For this review, take the finished solid that the model builds, in its own axes (mm). Give positions to 0.01 mm unless a question says otherwise; leave off trailing zeros. Write each loop counter-clockwise with the first axis right and the second up, starting at its lowest first coordinate (ties: lowest second). Pieces come first, ordered by that corner, then holes. Notation, with made-up numbers: M -27.5,-13 L 17.5,-13 A14 cw 17.5,-1 Z; hole C 68.25,62.5 d6. An arc over 180 degrees is marked long. Answer as a JSON object with one key per item and string values. Group by question number.
Autodesk Inventor part; units mm, degrees
ref_plane "YZ Plane" through (0, 0, 0) normal (1, 0, 0) x (0, 1, 0)
ref_plane "XZ Plane" through (0, 0, 0) normal (0, 1, 0) x (-1, 0, 0)
ref_plane "XY Plane" through (0, 0, 0) normal (0, 0, 1) x (1, 0, 0)
sketch "スケッチ1" plane through (0, 0, 0) normal (0, 0, 1) x (1, 0, 0)
  circle A0 centre (0, 0) radius 67.5
  dimension "d0" = 135
extrude "プレート1" add sketch "スケッチ1" along normal blind 2
sketch "スケッチ2" plane through (0, 0, 2) normal (0, 0, 1) x (1, 0, 0)
  circle A0 centre (0, 0) radius 38.5
  dimension "d2" = 77
extrude "押し出し1" cut sketch "スケッチ2" against normal through all
sketch "スケッチ3" plane through (0, 0, 2) normal (0, 0, 1) x (1, 0, 0)
  circle A0 centre (0, 0) radius 62.5
  point P0 (16.1762, 60.3704)
  point P1 (-16.1762, 60.3704)
  point P2 (-44.1942, 44.1942)
  point P3 (-60.3704, 16.1762)
  point P4 (-60.3704, -16.1762)
  point P5 (-44.1942, -44.1942)
  point P6 (-16.1762, -60.3704)
  point P7 (16.1762, -60.3704)
  point P8 (44.1942, -44.1942)
  point P9 (60.3704, -16.1762)
  point P10 (60.3704, 16.1762)
  point P11 (44.1942, 44.1942)
  dimension "d5" = 125
  dimension "d8" = 360
  dimension "d36" = 0
hole "穴1" at (16.1762, 60.3704, 2) at (-16.1762, 60.3704, 2) at (-44.1942, 44.1942, 2) at (-60.3704, 16.1762, 2) at (-60.3704, -16.1762, 2) at (-44.1942, -44.1942, 2) at (-16.1762, -60.3704, 2) at (16.1762, -60.3704, 2) at (44.1942, -44.1942, 2) at (60.3704, -16.1762, 2) at (60.3704, 16.1762, 2) at (44.1942, 44.1942, 2) direction (0, 0, -1) diameter 4.5 end through all
sketch "スケッチ4" plane through (0, 0, 2) normal (0, 0, 1) x (1, 0, 0)
  circle A0 centre (0, 0) radius 49
  point P0 (-34.6482, 34.6482)
  point P1 (-34.6482, -34.6482)
  point P2 (34.6482, -34.6482)
  point P3 (34.6482, 34.6482)
  dimension "d17" = 98
  dimension "d20" = 360
  dimension "d29" = 0
hole "穴2" at (-34.6482, 34.6482, 2) at (-34.6482, -34.6482, 2) at (34.6482, -34.6482, 2) at (34.6482, 34.6482, 2) direction (0, 0, -1) diameter 4.5 end through all
sketch "スケッチ6" plane through (0, 0, 0) normal (0, 0, -1) x (-1, 0, 0)
  circle A0 centre (0, 0) radius 37.5
  line L0 (-4.75, -42.3) -> (4.75, -42.3)
  line L1 (-4.75, -37.5) -> (4.75, -37.5)
  circle A1 centre (0, -37.5) radius 4.8
  point P0 (-4.75, -51.1)
  point P1 (4.75, -51.1)
  dimension "d37" = 75
  dimension "d38" = 9.5
  dimension "d39" = 8.8
  dimension "d40" = 13.6
  dimension "d41" = 4.75
hole "穴3" at (4.75, -51.1, 0) at (-4.75, -51.1, 0) direction (0, 0, 1) diameter 2.4 end through all
equation "\"d15\" = Thickness"
equation "\"d27\" = Thickness"
equation "\"d47\" = Thickness"
equation "\"d1\" = Thickness"
equation "\"BendRadius\" = Thickness"
equation "\"BendReliefWidth\" = Thickness"
equation "\"BendReliefDepth\" = 0.5 * Thickness"
equation "\"CornerReliefSize\" = 4 * Thickness"
equation "\"MinimumRemnant\" = 2 * Thickness"
equation "\"TransitionRadius\" = BendRadius"
equation "\"JacobiRadiusSize\" = BendRadius"
equation "\"GapSize\" = Thickness"
properties part number "unit-j2-plate1" material "CFRP"
Item 1: Draft analysis for pull direction X (two halves, no side actions). For faces 1 (the cylindrical face through (-53.57, 41.07, 0.99)), 2 (the flat face through (29, -29, 2)), 3 (the cylindrical face through (15.5, 58.224, 0.986)), state which applies: released by +X, released by -X, zero draft, split by the parting line, or undercut.
Item 2: Consider section A-A (x = 0). Give the boundary of the cut face in (y, z), plus the area to 3 significant figures.
Item 3: Consider section D-D (y = 54). Give the boundary of the cut face in (x, z).
Item 4: To check wall thickness, follow probe 1 along X at (y, z) = (45.5, 0.45); probe 2 along X at (y, z) = (-51, 0.9); probe 3 along Y at (x, z) = (16, 1.35). State the ranges of each line that lie inside material, in increasing order.
Item 5: Consider section C-C (z = 1.5). State how many separate pieces and enclosed holes the cut face has, plus the area to 3 significant figures.
Item 6: Insertion check: P1, Ø6, axis at x = -44.19, y = 44.19, coming from the -Z side; P2, Ø2.5, axis at x = -44.19, y = -44.19, coming from the +Z side. Each pin has a flat end and moves straight along its axis. Give the tip position at first contact, or say it passes through.
Result set:
{
 "1": {"face 1": "split by the parting line", "face 2": "zero draft", "face 3": "undercut"},
 "2": {"outline": "M -67.5,0 L -38.5,0 L -38.5,2 L -67.5,2 Z; M 38.5,0 L 67.5,0 L 67.5,2 L 38.5,2 Z", "area": "116 mm^2"},
 "3": {"outline": "M -40.5,0 L 40.5,0 L 40.5,2 L -40.5,2 Z"},
 "4": {"probe 1": "x = -49.86 to -46.03, -42.36 to 42.36, 46.03 to 49.86", "probe 2": "x = -44.22 to -5.95, -3.55 to 3.55, 5.95 to 44.22", "probe 3": "y = -65.58 to -62.61, -58.13 to -35.02, 35.02 to 58.13, 62.61 to 65.58"},
 "5": {"separate pieces": "1", "enclosed holes": "19", "area": "9,390 mm^2"},
 "6": {"P1": "stops at z = 0", "P2": "passes through"}
}
